Read the model definition and answer for the solid it produces. Units are mm, in the model's axes. Coordinates: 2 decimals unless noted, no trailing zeros. Loops run counter-clockwise (first coordinate to the right, second up) from the corner with the lowest first, then second, coordinate; pieces in that order, holes last. Notation, with made-up numbers: (23.5, 48.5) -> (54.5, 48.5) arc R21 ccw to (54.5, 82.5) -> close; hole circle Ø10 at (32.25, 88). An arc over 180 degrees is marked (long way). One line per question, with ' | ' between items. Start each with the question number.
```python
from build123d import *

# Parameters (mm, degrees)
SKETCH1_R           = 20.32
BOSS_EXTRUDE1_DEPTH = 6.35


with BuildPart() as part:
    # Sketch1 → Boss-Extrude1 (new body)
    with BuildSketch(Plane(origin=(0, 0, 0), x_dir=(1, 0, 0), z_dir=(0, 1, 0))):
        Polygon((-38.1, -38.1), (38.1, -38.1), (38.1, 38.1), (-38.1, 38.1), (-38.1, 24.13), (-46.2026, 24.13), (-46.2026, 20.447), (-44.0944, 20.447), (-44.0944, 17.78), (-51.9684, 17.78), (-51.9684, 20.447), (-49.8602, 20.447), (-49.8602, 24.13), (-57.9628, 24.13), (-57.9628, 9.9314), (-38.1, 9.9314), (-38.1, -9.9314), (-57.9628, -9.9314), (-57.9628, -24.13), (-49.8602, -24.13), (-49.8602, -20.447), (-51.9684, -20.447), (-51.9684, -17.78), (-44.0944, -17.78), (-44.0944, -20.447), (-46.2026, -20.447), (-46.2026, -24.13), (-38.1, -24.13), align=None)
        Circle(SKETCH1_R, mode=Mode.SUBTRACT)
    extrude(amount=-BOSS_EXTRUDE1_DEPTH)


solid = part.part
```
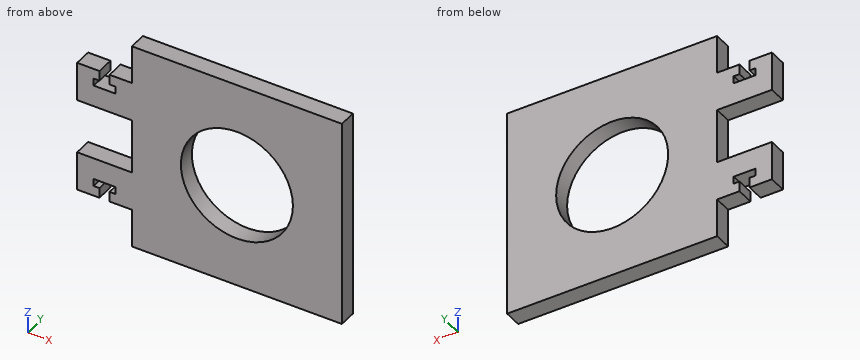
(1) Find the intervals of material crossed by probe 1 along X at (y, z) = (-1.5, 21.5); probe 2 along Z at (x, y) = (-40.5, -3.5); probe 3 along X at (y, z) = (-4.5, 18.5), in increasing order. Write a range as from..to.
(2) Section B-B on z = 0 is taken. Write down the section's boundary in (x, y), plus the area to 3 significant figures.
(3) Each of these flat-tipped pins is pushed along its axis until it touches: pin 1 Ø1.9 at (x, y) = (-41, -3.5) entering from +Z; pin 2 Ø1.7 at (x, y) = (-44.5, -3) entering from -Z; pin 3 Ø8 at (x, z) = (6.5, 24.5) entering from +Y; pin 4 Ø8 at (x, z) = (-46.5, -5) entering from +Y. Where does it stop, or does it pass through?
(4) Section A-A on x = 0 is taken. Write down the section's boundary in (y, z), plus the area to 3 significant figures.
Working result:
1) probe 1: x = -57.96..-49.86, -46.2..38.1 | probe 2: z = -24.13..-9.93, 9.93..24.13 | probe 3: x = -57.96..-51.97, -44.09..-8.41, 8.41..38.1
2) outline: (-38.1, -6.35) -> (-20.32, -6.35) -> (-20.32, 0) -> (-38.1, 0) -> close; (20.32, -6.35) -> (38.1, -6.35) -> (38.1, 0) -> (20.32, 0) -> close | area: 226 mm2
3) pin 1: stops at z = 24.13 | pin 2: stops at z = -24.13 | pin 3: stops at y = 0 | pin 4: passes through
4) outline: (-6.35, -38.1) -> (0, -38.1) -> (0, -20.32) -> (-6.35, -20.32) -> close; (-6.35, 20.32) -> (0, 20.32) -> (0, 38.1) -> (-6.35, 38.1) -> close | area: 226 mm2
